Check sheet for the modelled part. Datum: model origin and axes. Units: mm. A direction names the side the tool comes from. Round coordinates to 2 decimals unless told otherwise and drop trailing zeros. Answer in a Markdown table with one row per item.
```python
from build123d import *

# Parameters (mm, degrees)
SKETCH1_R           = 2
BOSS_EXTRUDE1_DEPTH = 450
SKETCH2_R           = 4.1
CUT_EXTRUDE1_DEPTH  = 451.325671043


with BuildPart() as part:
    # Sketch1 → Boss-Extrude1 (new body)
    with BuildSketch(Plane.XY):
        Polygon((10, 10), (10, 4.610379336), (8.2, 3.1), (8.2, 5.5), (6.560660172, 5.5), (3.9, 2.839339828), (3.9, 0.519615242), (3.6, 0), (3.9, -0.519615242), (3.9, -2.839339828), (6.560660172, -5.5), (8.2, -5.5), (8.2, -3.1), (10, -4.610379336), (10, -10), (4.610379336, -10), (3.1, -8.2), (5.5, -8.2), (5.5, -6.560660172), (2.839339828, -3.9), (0.519615242, -3.9), (0, -3.6), (-0.519615242, -3.9), (-2.839339828, -3.9), (-5.5, -6.560660172), (-5.5, -8.2), (-3.1, -8.2), (-4.610379336, -10), (-10, -10), (-10, -4.610379336), (-8.2, -3.1), (-8.2, -5.5), (-6.560660172, -5.5), (-3.9, -2.839339828), (-3.9, -0.519615242), (-3.6, 0), (-3.9, 0.519615242), (-3.9, 2.839339828), (-6.560660172, 5.5), (-8.2, 5.5), (-8.2, 3.1), (-10, 4.610379336), (-10, 10), (-4.610379336, 10), (-3.1, 8.2), (-5.5, 8.2), (-5.5, 6.560660172), (-2.839339828, 3.9), (-0.519615242, 3.9), (0, 3.6), (0.519615242, 3.9), (2.839339828, 3.9), (5.5, 6.560660172), (5.5, 8.2), (3.1, 8.2), (4.610379336, 10), align=None)
        Circle(SKETCH1_R, mode=Mode.SUBTRACT)
    extrude(amount=BOSS_EXTRUDE1_DEPTH)

    # Sketch2 → Cut-Extrude1 (cut, through all)
    with BuildSketch(Plane(origin=(3.9, 0, 0), x_dir=(0, 0, -1), z_dir=(1, 0, 0))):
        with Locations(Location((-380, 0, 0), (0, 0, 136.169927123))):
            Circle(SKETCH2_R)
        with Locations(Location((-70, 0, 0), (0, 0, 136.169927123))):
            Circle(SKETCH2_R)
    extrude(amount=-CUT_EXTRUDE1_DEPTH, mode=Mode.SUBTRACT)


solid = part.part
```
(1) Depth check by flat-ended pin: pin 1 Ø0.7 at (y, z) = (-1.5, 425.5) entering from -X; pin 2 Ø4 at (x, y) = (6, 7.5) entering from -Z; pin 3 Ø2.5 at (x, z) = (-2, 39) entering from -Y; pin 4 Ø0.7 at (x, z) = (1.5, 20) entering from -Y. Enter the tip coordinate at first touch or a pass-through.
Solutions:
| item | result |
|---|---|
| pin 1 | x = -3.9 |
| pin 2 | z = 0 |
| pin 3 | y = -8.38 |
| pin 4 | y = -3.9 |
(2) Draft check along Y on faces 1 (the cylindrical face through (-0.664, 2.272, 66.587)), 2 (the flat face through (0.1, 2.4, 0)). Enter one of: pulls with the +Y half, pulls with the -Y half, needs draft (parallel to the pull), parting line crosses it, or undercut.
Solutions:
| item | result |
|---|---|
| face 1 | undercut |
| face 2 | needs draft |
(3) Tool access check on faces 3 (the flat face through (0.1, 2.4, 450)), 4 (the cylindrical face through (-0.664, 2.272, 376.587)). Record the directions out of +Z, -Z, +X, -X, +Y, -Y that give a thin tool (end or side, any length) a straight path to the whole face; none if there is none.
Solutions:
| item | result |
|---|---|
| face 3 | +Z, +X, -X, +Y, -Y |
| face 4 | -X |
(4) Scan lines: probe 1 along X at (y, z) = (0, 295); probe 2 along Z at (x, y) = (3.5, -0.25); probe 3 along Y at (x, z) = (-7, 237). Record each from-to range of solid material in increasing order. Write a range as from..to.
Solutions:
| item | result |
|---|---|
| probe 1 | -3.6..-2, 2..3.6 |
| probe 2 | 0..65.91, 74.09..375.91, 384.09..450 |
| probe 3 | -10..-5.5, 5.5..10 |
